from build123d import *

# Parameters (mm, degrees)
F0_W     = 3.175
F0_H     = 101.6
F1_DEPTH = 228.6
F2_DEPTH = 236.22
F0_W_2   = 21.717
F3_DEPTH = 3.175
F4_W     = 76.0733831866
F4_H     = 5.55625
F5_DEPTH = 3.175


# Not quite as in the source:
# - the program builds the solid bodies; features that only make, move or delete a surface that nothing else refers to are left out


with BuildPart() as f1:
    # F0 (on Top) → F1 (new body)
    with BuildSketch(Plane.XY):
        with Locations((36.5125, -2.4078887083)):
            Rectangle(F0_W, F0_H)
    extrude(amount=F1_DEPTH)

    # F0 (on Top) → F2 (join)
    with BuildSketch(Plane.XY):
        Polygon((-34.925, 48.3921112917), (-13.208, 48.3921112917), (13.208, 48.3921112917), (34.925, 48.3921112917), (38.1, 48.3921112917), (38.1, 51.5671112917), (-38.1, 51.5671112917), (-38.1, 48.3921112917), align=None)
        Polygon((-34.925, -53.2078887083), (-34.925, 48.3921112917), (-38.1, 48.3921112917), (-38.1, -53.3400028944), align=None)
        Polygon((13.208, -53.2078887083), (-13.208, -53.2078887083), (-34.925, -53.2078887083), (-38.1, -53.3400028944), (-37.9733831866, -56.3828887083), (38.1, -56.3828887083), (38.1, -53.2078887083), (34.925, -53.2078887083), align=None)
        with Locations((36.5125, -2.4078887083)):
            Rectangle(F0_W, F0_H)
    extrude(amount=F2_DEPTH)

    # F0 (on Top) → F3 (join)
    with BuildSketch(Plane.XY):
        with Locations((-24.0665, -2.4078887083)):
            Rectangle(F0_W_2, F0_H)
        with Locations((24.0665, -2.4078887083)):
            Rectangle(F0_W_2, F0_H)
    extrude(amount=F3_DEPTH)

    # F4 (on face) → F5 (cut)
    with BuildSketch(Plane.XZ.offset(56.3828887083)):
        with Locations((0.0633084067, 2.778125)):
            Rectangle(F4_W, F4_H)
    extrude(amount=-F5_DEPTH, mode=Mode.SUBTRACT)


solid = f1.part
Input: part model. Units: mm. Frame: model coordinates. A direction names the side the tool comes from. Coordinates: 2 decimals unless noted, no trailing zeros. Loops run counter-clockwise (first coordinate to the right, second up) from the corner with the lowest first, then second, coordinate; pieces in that order, holes last.
Q1. Set-up query: faces 4 (the face through (-38.1, 0, 116)), 5 (the face through (25, -53.208, 2)), 6 (the face through (-24, -2, 3.175)), 7 (the face through (0, -53.208, 119)). Return all of +Z, -Z, +X, -X, +Y, -Y with unobstructed straight access to the full face (end or side cutting, diameter ignored); none if empty.
Q2. Cut plane C-C (y = -48). Output: boundary loops of the cut face in (x, z) (3 decimals).
Q3. Contact query for flat-ended pins moving along their axis: pin 1 (3 mm diameter, centred on x = 26, y = 35, fed in from +Z) (3 decimals); pin 2 (3 mm diameter, centred on x = -30, y = 31, fed in from -Z); pin 3 (3.5 mm diameter, centred on y = -55, z = 2, fed in from +X); pin 4 (1.6 mm diameter, centred on x = -0.5, y = -54.5, fed in from -Z). Output: stop coordinate, or through.
Q4. Draft query along Y for faces 1 (the face through (24, -2, 3.175)), 2 (the face through (-34.925, -3, 118)), 3 (the face through (-26, -53.208, 2)). Return one class per face: +Y half, -Y half, draft (parallel to the pull), parting line (faces both ways), or undercut.
Q5. Material intervals for line 1 (Y direction, x = -33.5, z = 65.5); line 2 (X direction, y = -14, z = 103) (3 decimals); line 3 (Z direction, x = 29, y = 45.5) (3 decimals), sorted ascending.
Q6. Cut plane A-A (z = 220). Output: boundary loops of the cut face in (x, y) (3 decimals), then the cut area to 3 significant figures.
Q7. Cut plane D-D (x = 8.5). Output: boundary loops of the cut face in (y, z), then the cut area to 3 significant figures.
Q8. Cut plane B-B (x = 21). Output: boundary loops of the cut face in (y, z) (3 decimals), then the cut area to 3 significant figures.
Working result:
1. face 4: +Z, -Z, -X, +Y, -Y
1. face 5: -Z, +X, -Y
1. face 6: +Z, -Y
1. face 7: +Z
2. outline: (-38.1, 0) - (-13.208, 0) - (-13.208, 3.175) - (-34.925, 3.175) - (-34.925, 236.22) - (-38.1, 236.22) - close; (13.208, 0) - (38.1, 0) - (38.1, 236.22) - (34.925, 236.22) - (34.925, 3.175) - (13.208, 3.175) - close
3. pin 1: stops at z = 3.175
3. pin 2: stops at z = 0
3. pin 3: stops at x = -37.97
3. pin 4: stops at z = 5.56
4. face 1: draft
4. face 2: undercut
4. face 3: -Y half
5. line 1: y = -56.38 to -53.21, 48.39 to 51.57
5. line 2: x = -38.1 to -34.925, 34.925 to 38.1
5. line 3: z = 0 to 3.175
6. outline: (-38.1, -53.34) - (-37.973, -56.383) - (38.1, -56.383) - (38.1, 51.567) - (-38.1, 51.567) - close; hole (-34.925, -53.208) - (34.925, -53.208) - (34.925, 48.392) - (-34.925, 48.392) - close
6. area: 1,130 mm2
7. outline: (-56.38, 5.56) - (-53.21, 5.56) - (-53.21, 236.22) - (-56.38, 236.22) - close; (48.39, 0) - (51.57, 0) - (51.57, 236.22) - (48.39, 236.22) - close
7. area: 1,480 mm2
8. outline: (-56.383, 5.556) - (-53.208, 5.556) - (-53.208, 236.22) - (-56.383, 236.22) - close; (-53.208, 0) - (51.567, 0) - (51.567, 236.22) - (48.392, 236.22) - (48.392, 3.175) - (-53.208, 3.175) - close
8. area: 1,800 mm2
